Part print with two shaded views. Sizes in mm from the minimum x, y, z corner. Coordinates: 2 decimals unless noted, no trailing zeros. Order: outer loops, then holes, each group sorted by start corner. A loop starts at its lowest first (then second) coordinate and runs counter-clockwise, first axis right, second up. Notation, with made-up numbers: (-30.5, 7) - (28.5, 7) arc R22 ccw to (28.5, 22) - close; hole circle Ø1 at (13, -15.5). An arc over 180 degrees is marked (long way). One line per item, written item: value.
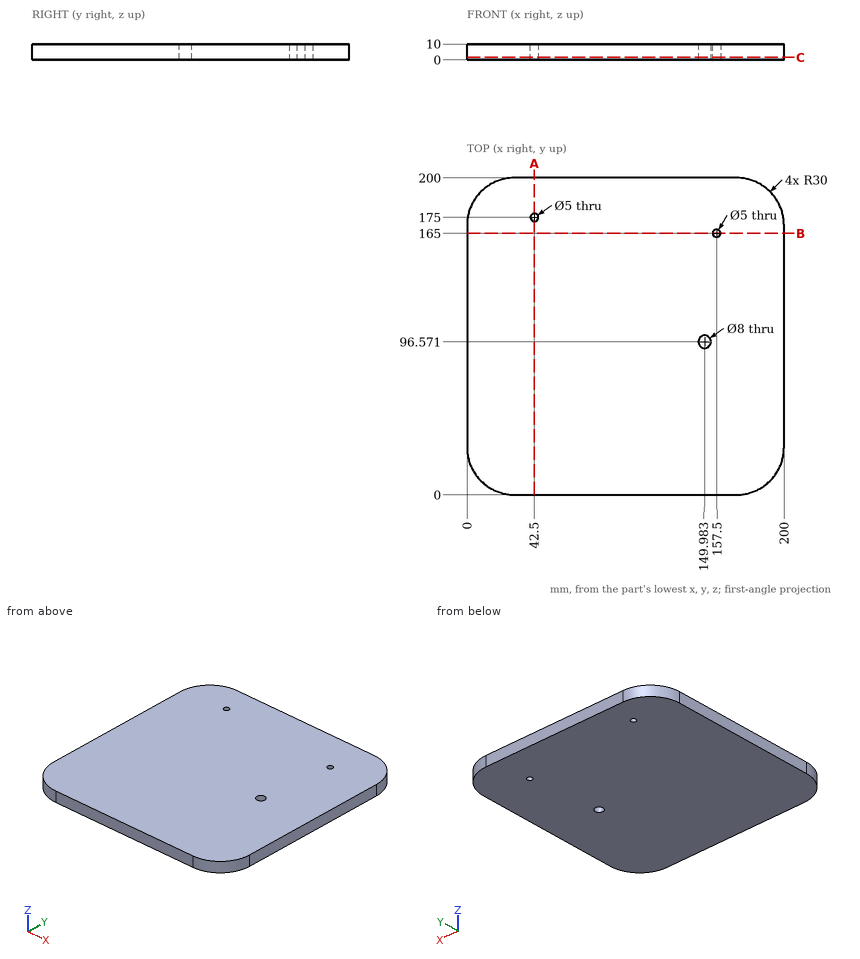
1. Band-saw the part on B-B, the plane y = 165. Give the cut face in (x, z).
Values found:
outline: (0, 0) - (155, 0) - (155, 10) - (0, 10) - close; (160, 0) - (200, 0) - (200, 10) - (160, 10) - close
2. Band-saw the part on A-A, the plane x = 42.5. Give the cut face in (y, z).
Values found:
outline: (0, 0) - (172.5, 0) - (172.5, 10) - (0, 10) - close; (177.5, 0) - (200, 0) - (200, 10) - (177.5, 10) - close
3. Band-saw the part on C-C, the plane z = 1.5. Give the cut face in (x, y).
Values found:
outline: (0, 30) arc R30 ccw to (30, 0) - (170, 0) arc R30 ccw to (200, 30) - (200, 170) arc R30 ccw to (170, 200) - (30, 200) arc R30 ccw to (0, 170) - close; hole circle Ø5 at (42.5, 175); hole circle Ø8 at (149.98, 96.57); hole circle Ø5 at (157.5, 165)
4. Probe line 1 along X through (y, z) = (165, 5); line 2 along Y through (x, z) = (157.5, 7.25); line 3 along Y through (x, z) = (153.5, 5) (1 decimal). List the from-to ranges inside material, lowest first.
Values found:
line 1: x = 0 to 155, 160 to 200
line 2: y = 0 to 162.5, 167.5 to 200
line 3: y = 0 to 94.7, 98.5 to 200
